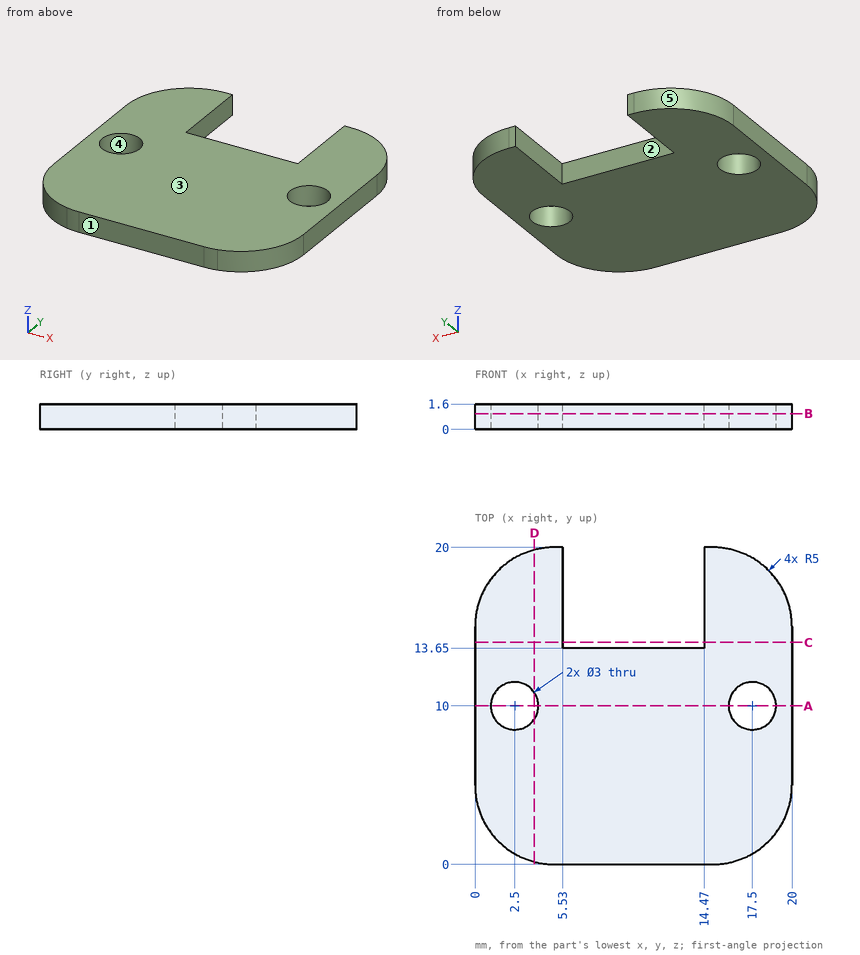
Job drawing, mm, ordinate dimensions from the low corner. One solid piece. A direction names the side the tool comes from. Give positions to 0.01 mm unless a question says otherwise; leave off trailing zeros. Loops run counter-clockwise (first coordinate to the right, second up) from the corner with the lowest first, then second, coordinate; pieces in that order, holes last. Notation, with made-up numbers: M 68,-35.75 L 120,-35.75 A22 cw 120,-4.75 Z; hole C 62.25,-9.5 d7. An arc over 180 degrees is marked long. Put each result on its own line as item: value. Start each with the question number.
1) Saw through at A-A (y = 10). List the corners of the cut face in (x, z).
2) Probe probe 1 along X at (y, z) = (10, 1.25); probe 2 along X at (y, z) = (14, 0.4); probe 3 along X at (y, z) = (8.75, 0.8). List the from-to ranges inside material, lowest first.
3) 3-axis set-ups, long thin cutter, end or side, ignore diameter. For the marked faces 1 and 2: which of +Z, -Z, +X, -X, +Y, -Y reach the whole face in a straight line?
4) Saw through at C-C (y = 14). List the corners of the cut face in (x, z).
5) Pull direction X, two halves, no side cores. Call the marked faces 3, 4 and 5: +X half, -X half, draft (parallel to the pull), parting line (faces both ways), or undercut.
6) Saw through at B-B (z = 1). List the corners of the cut face in (x, y), then the cut area to 3 significant figures.
7) Saw through at D-D (x = 3.75). List the corners of the cut face in (y, z), then the cut area to 3 significant figures.
8) Flat gauge pins, fed straight in: pin 1 (0.5 mm diameter, centred on y = 18, z = 1, fed in from +X); pin 2 (4 mm diameter, centred on x = 17.5, y = 10, fed in from +Z). Where does each tip first touch, or does it go through?
Numbers:
1. outline: M 0,0 L 1,0 L 1,1.6 L 0,1.6 Z; M 4,0 L 16,0 L 16,1.6 L 4,1.6 Z; M 19,0 L 20,0 L 20,1.6 L 19,1.6 Z
2. probe 1: 0 to 1, 4 to 16, 19 to 20
2. probe 2: 0 to 5.53, 14.47 to 20
2. probe 3: 0 to 1.67, 3.33 to 16.67, 18.33 to 20
3. face 1: +Z, -Z, +X, -X, -Y
3. face 2: +Z, -Z, +Y
4. outline: M 0,0 L 5.53,0 L 5.53,1.6 L 0,1.6 Z; M 14.47,0 L 20,0 L 20,1.6 L 14.47,1.6 Z
5. face 3: draft
5. face 4: undercut
5. face 5: -X half
6. outline: M 0,5 A5 ccw 5,0 L 15,0 A5 ccw 20,5 L 20,15 A5 ccw 15,20 L 14.47,20 L 14.47,13.65 L 5.53,13.65 L 5.53,20 L 5,20 A5 ccw 0,15 Z; hole C 2.5,10 d3; hole C 17.5,10 d3
6. area: 308 mm^2
7. outline: M 0.16,0 L 9.17,0 L 9.17,1.6 L 0.16,1.6 Z; M 10.83,0 L 19.84,0 L 19.84,1.6 L 10.83,1.6 Z
7. area: 28.8 mm^2
8. pin 1: x = 19.18
8. pin 2: z = 1.6
